Source: CAD feature listing. Evaluate the final solid. Frame: model axes, mm. Face numbers are marked on the shaded views. A direction names the side the tool comes from. Round coordinates to 2 decimals unless told otherwise and drop trailing zeros. Order: outer loops, then holes, each group sorted by start corner. A loop starts at its lowest first (then second) coordinate and runs counter-clockwise, first axis right, second up. Notation, with made-up numbers: (24, 76.5) -> (61, 76.5) arc R21 cw to (61, 80.5) -> close; hole circle Ø9 at (31.25, 9). An arc over 180 degrees is marked (long way). Answer as CSV lines item,"result".
from build123d import *

# Parameters (mm, degrees)
PAD_DEPTH     = 13
SKETCH001_R   = 39
PAD001_DEPTH  = 5
SKETCH002_R   = 36.5
POCKET_DEPTH  = 15.75
PAD002_DEPTH  = 15
SKETCH004_W   = 2.317019
SKETCH004_H   = 4.5
SKETCH004_W_2 = 2.064228
PAD003_DEPTH  = 6


with BuildPart() as part:
    # Sketch → Pad (new body)
    with BuildSketch(Plane.XY):
        with BuildLine():
            Line((8.98454, 37.950995), (28.389288, 33.357104))
            ThreePointArc((39, 19.941115), (36.026709, 28.493542), (28.389288, 33.357104))
            Line((39, 0), (39, 19.941115))
            ThreePointArc((38.00467, -8.754718), (38.750368, -4.405558), (39, 0))
            Line((38.00467, -8.754718), (34.750723, -22.880263))
            ThreePointArc((14.495489, -39), (27.438831, -34.478227), (34.750723, -22.880263))
            Line((4e-06, -39), (14.495489, -39))
            Line((4e-06, -39), (-14.495489, -39))
            ThreePointArc((-34.750723, -22.880263), (-27.438831, -34.478227), (-14.495489, -39))
            Line((-38.00467, -8.754718), (-34.750723, -22.880263))
            ThreePointArc((-39, 0), (-38.750368, -4.405558), (-38.00467, -8.754718))
            Line((-39, 0), (-39, 19.941115))
            ThreePointArc((-28.389288, 33.357104), (-35.611883, 28.165455), (-39, 19.941115))
            Line((-8.98454, 37.950995), (-28.389288, 33.357104))
            ThreePointArc((8.98454, 37.950995), (0, 39), (-8.98454, 37.950995))
        make_face()
    extrude(amount=PAD_DEPTH)

    # Sketch001 (on Face17 of Pad) → Pad001 (join)
    with BuildSketch(Plane.XY.offset(13)):
        Circle(SKETCH001_R)
    extrude(amount=PAD001_DEPTH)

    # Sketch002 (on Face22 of Pad001) → Pocket (cut)
    with BuildSketch(Plane.XY.offset(18)):
        Circle(SKETCH002_R)
    extrude(amount=-POCKET_DEPTH, mode=Mode.SUBTRACT)

    # Sketch003 (on Face22 of Pocket) → Pad002 (join)
    with BuildSketch(Plane.XY.offset(18)):
        with BuildLine():
            ThreePointArc((-36.942523, 12.5), (-38.995202, 0), (-36.942523, -12.5))
            Line((-36.942523, -12.5), (-34.292856, -12.5))
            ThreePointArc((-34.292856, 12.5), (-36.5, 0), (-34.292856, -12.5))
            Line((-36.942523, 12.5), (-34.292856, 12.5))
        make_face()
        with BuildLine():
            ThreePointArc((34.292856, -12.5), (36.505526, 0), (34.292856, 12.5))
            Line((34.292856, 12.5), (36.942523, 12.5))
            ThreePointArc((36.942523, -12.5), (39, 0), (36.942523, 12.5))
            Line((34.292856, -12.5), (36.942523, -12.5))
        make_face()
    extrude(amount=PAD002_DEPTH)

    # Sketch004 (on Face35 of Pad002) → Pad003 (join)
    with BuildSketch(Plane.XY.offset(33)):
        with Locations((-36.589095, 0)):
            Rectangle(SKETCH004_W, SKETCH004_H)
        with Locations((36.468061, 0)):
            Rectangle(SKETCH004_W_2, SKETCH004_H)
    extrude(amount=-PAD003_DEPTH)


solid = part.part
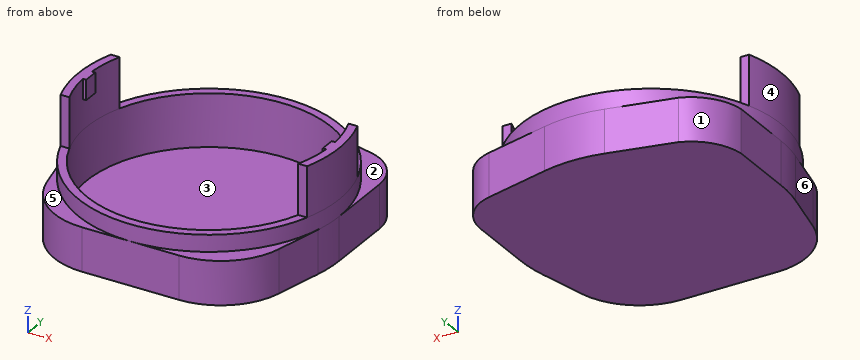
1. Pin query (flat end, axial travel): pin 1 (1.5 mm diameter, centred on x = 12, y = 20.5, fed in from -Z); pin 2 (4 mm diameter, centred on y = -15.5, z = 4, fed in from +X); pin 3 (0.8 mm diameter, centred on x = -35, z = 25.5, fed in from +Y); pin 4 (12 mm diameter, centred on x = -29, y = 6, fed in from +Z). Return the tip coordinate at first contact, or that it passes through.
Results below:
pin 1,"z = 0"
pin 2,"x = 36.91"
pin 3,"y = 12.5"
pin 4,"z = 2.25"
2. Section query D-D on z = 15. Return loops of the section in (x, y).
Results below:
outline,"circle Ø78 at (0, 0); hole circle Ø73 at (0, 0)"
3. Section query A-A on z = 25.5. Return loops of the section in (x, y), and give its area (3 significant figures).
Results below:
outline,"(-36.94, -12.5) -> (-34.29, -12.5) arc R36.5 cw to (-34.29, 12.5) -> (-36.94, 12.5) arc R39.09 ccw to start; (34.29, -12.5) -> (36.94, -12.5) arc R39 ccw to (36.94, 12.5) -> (34.29, 12.5) arc R36.41 cw to start"
area,"127 mm2"
4. Mould query, pull axis X, two halves, no side actions, for the marked faces 1, 2 and 3. Classes: released by +X, released by -X, zero draft, split by the parting line, or undercut.
Results below:
face 1,"released by -X"
face 2,"zero draft"
face 3,"undercut"
5. Reachability of the marked faces 4, 5 and 6 from +Z, -Z, +X, -X, +Y, -Y: full face, straight path, thin tool, end or side. Return the list, or none.
Results below:
face 4,"+Z, -X"
face 5,"+Z, -X, -Y"
face 6,"+Z, -Z, -X, -Y"
6. Line query: L1, parallel to Y at x = 0, z = 12.25; L2, parallel to Z at x = -26, y = 1; L3, parallel to X at y = 26.5, z = 12. Output: solid intervals per line, ascending. Write a range as [from, to].
Results below:
L1,"[-39, -36.5], [36.5, 39]"
L2,"[0, 2.25]"
L3,"[-36.77, -25.1], [25.1, 37.34]"
